```python
from build123d import *


with BuildPart() as part:
    # Sketch1 → Revolve1 (revolve)
    with BuildSketch(Plane.XY, mode=Mode.PRIVATE) as revolve1_sk:
        with BuildLine():
            ThreePointArc((5, -3.31662479), (5.744562647, -1.732050808), (6, 0))
            Line((6, 0), (6, 35))
            ThreePointArc((6, 35), (6.002835942, 36.115484437), (4.893341951, 36))
            ThreePointArc((4.893341951, 36), (4.754229922, 35.479474613), (5, 35))
            Line((5, 35), (5, 0))
            ThreePointArc((5, 0), (3.535533906, -3.535533906), (0, -5))
            Line((0, -5), (0, -6))
            ThreePointArc((0, -6), (2.837274331, -5.286764074), (5, -3.31662479))
        make_face()
    revolve(revolve1_sk.sketch.rotate(Axis((0, 0, 0), (0, 1, 0)), 90), axis=Axis((0, 0, 0), (0, 1, 0)))


solid = part.part
```
Model file for the job. Use its own axes, mm. Coordinates: 2 decimals unless noted, no trailing zeros. Loops run counter-clockwise (first coordinate to the right, second up) from the corner with the lowest first, then second, coordinate; pieces in that order, holes last. Notation, with made-up numbers: (68, -32.75) - (113, -32.75) arc R17 cw to (113, -26.75) - close; hole circle Ø7 at (-19, -19). An arc over 180 degrees is marked (long way). Answer as a JSON object with one key per item and string values. Group by question number.
(1) Probe line 1 along X through (y, z) = (8.5, 0); line 2 along Z through (x, y) = (-0.25, 12); line 3 along Z through (x, y) = (-3, 32). List the from-to ranges inside material, lowest first.
(2) Cut at A-A (y = 21). Give the cut face in (x, z).
(3) Two-plate mould, pull along Z, no slides. Class faces 1 (the face through (-1.802, 17.745, -5.723)), 2 (the face through (0, 17, 5)): released by +Z, released by -Z, zero draft, split by the parting line, or undercut.
(4) Flat gauge pins, fed straight in: pin 1 (6 mm diameter, centred on x = -3.5, y = 20.5, fed in from -Z); pin 2 (4 mm diameter, centred on x = 0, y = 8, fed in from +Z); pin 3 (5 mm diameter, centred on x = -3.5, z = 1.5, fed in from -Y). Where does each tip first touch, or does it go through?
Geometry says:
{
 "1": {"line 1": "x = -6 to -5, 5 to 6", "line 2": "z = -5.99 to -4.99, 4.99 to 5.99", "line 3": "z = -5.2 to -4, 4 to 5.2"},
 "2": {"outline": "circle Ø12 at (0, 0); hole circle Ø10 at (0, 0)"},
 "3": {"face 1": "split by the parting line", "face 2": "undercut"},
 "4": {"pin 1": "stops at z = -5.98", "pin 2": "stops at z = 6", "pin 3": "stops at y = -5.86"}
}
